Could you check a few things on this model? Use its own coordinates, in mm. A direction names the side the tool comes from. Give positions to 0.01 mm unless a question says otherwise; leave off trailing zeros. Order: outer loops, then holes, each group sorted by start corner. A loop starts at its lowest first (then second) coordinate and runs counter-clockwise, first axis right, second up. Notation, with made-up numbers: M 35.25,60 L 46.25,60 A27 cw 46.25,77 Z; hole C -1,44.5 d1. An arc over 180 degrees is marked long. Use a Markdown table: item, result. Add a question column.
Item 1: For faces 3 (the face through (25, 1, 8)), 4 (the face through (-38, 14.616, 23)), 5 (the face through (38, -9, 38)), which set-ups out of +Z, -Z, +X, -X, +Y, -Y let a thin tool reach every point of the face, with its end or its side?
Item 2: If we mould it in two halves opening along X, with no side actions, what happens to faces 1 (the face through (-23.977, 1.055, 4.056)), 2 (the face through (-41, 0, 23))? For each: released by +X, released by -X, zero draft, split by the parting line, or undercut.
Item 3: Suppose I cut it at B-B on y = -7. Write out the boundary of the cut face in (x, z), plus the area to 3 significant figures.
Item 4: Suppose I cut it at D-D on y = -25.5. Write out the boundary of the cut face in (x, z).
Item 5: Suppose I cut it at A-A on x = 0. Write out the boundary of the cut face in (y, z) (3 decimals).
Item 6: Suppose I cut it at C-C on z = 25. Write out the boundary of the cut face in (x, y) (3 decimals).
Item 7: I'm going to push flat-ended pins straight in: pin 1 Ø5 at (x, z) = (-38, 26) entering from -Y; pin 2 Ø12 at (x, z) = (10, 19.5) entering from -Y; pin 3 Ø10 at (x, z) = (-17, 33.5) entering from -Y. Where does each tip first touch, or does it pass through?
Item 8: If I drill on L1, parallel to Y at x = 0, z = 5 (3 decimals); L2, parallel to Z at x = -7.5, y = 28.5; L3, parallel to Y at x = -13.5, z = 25.5, over which ranges is the centre line in solid material (lowest first)? Write a range as from..to.
from build123d import *

# Parameters (mm, degrees)
SKETCH1_R           = 42.875
BOSS_EXTRUDE1_DEPTH = 8
BOSS_EXTRUDE2_DEPTH = 30
SKETCH4_R           = 24
CUT_EXTRUDE1_DEPTH  = 20


with BuildPart() as part:
    # Sketch1 → Boss-Extrude1 (new body)
    with BuildSketch(Plane.XY):
        Circle(SKETCH1_R)
    extrude(amount=BOSS_EXTRUDE1_DEPTH)

    # Sketch2 → Boss-Extrude2 (add)
    with BuildSketch(Plane.XY.offset(8)):
        with BuildLine():
            ThreePointArc((38.725, 0), (0, -38.725), (-38.725, 0))
            Line((-38.725, 0), (-42.875, 0))
            ThreePointArc((-42.875, 0), (0, -42.875), (42.875, 0))
            ThreePointArc((42.875, 0), (7.419974343, 42.228066564), (-40.30678919, 14.616031274))
            Line((-40.30678919, 14.616031274), (-35.860803878, 14.616031274))
            ThreePointArc((-35.860803878, 14.616031274), (7.44701265, 38.002205562), (38.725, 0))
        make_face()
    extrude(amount=BOSS_EXTRUDE2_DEPTH)

    # Sketch4 → Cut-Extrude1 (cut)
    with BuildSketch(Plane.XY.offset(8)):
        Circle(SKETCH4_R)
    extrude(amount=-CUT_EXTRUDE1_DEPTH, mode=Mode.SUBTRACT)


solid = part.part
Findings below:
| question | item | result |
|---|---|---|
| 1 | face 3 | +Z |
| 1 | face 4 | +Z, -X |
| 1 | face 5 | +Z, +X, -X, +Y, -Y |
| 2 | face 1 | undercut |
| 2 | face 2 | zero draft |
| 3 | outline | M -42.3,0 L -22.96,0 L -22.96,8 L -38.09,8 L -38.09,38 L -42.3,38 Z; M 22.96,0 L 42.3,0 L 42.3,38 L 38.09,38 L 38.09,8 L 22.96,8 Z |
| 3 | area | 562 mm^2 |
| 4 | outline | M -34.47,0 L 34.47,0 L 34.47,38 L 29.14,38 L 29.14,8 L -29.14,8 L -29.14,38 L -34.47,38 Z |
| 5 | outline | M -42.875,0 L -24,0 L -24,8 L -38.725,8 L -38.725,38 L -42.875,38 Z; M 24,0 L 42.875,0 L 42.875,38 L 38.725,38 L 38.725,8 L 24,8 Z |
| 6 | outline | M -42.875,0 A42.875 ccw long -40.307,14.616 L -35.861,14.616 A38.725 cw long -38.725,0 Z |
| 7 | pin 1 | stops at y = -24.04 |
| 7 | pin 2 | stops at y = -42.69 |
| 7 | pin 3 | stops at y = -41.16 |
| 8 | L1 | y = -42.875..-24, 24..42.875 |
| 8 | L2 | z = 0..8 |
| 8 | L3 | y = -40.69..-36.3, 36.3..40.69 |
